```python
from build123d import *

# Parameters (mm, degrees)
PAD004_DEPTH    = 30
FILLET002_R     = 5
FILLET003_R     = 5
CHAMFER002_SIZE = 1


with BuildPart() as part:
    # Sketch006 → Pad004 (new body)
    with BuildSketch(Plane.YZ):
        Polygon((0, 0), (0, 80), (-5, 80), (-5, 121.25), (32.5, 121.25), (32.5, 116.25), (2.5, 116.25), (2.5, -36.25), (32.5, -36.25), (32.5, -41.25), (-5, -41.25), (-5, 0), align=None)
    extrude(amount=PAD004_DEPTH)

    # Fillet002
    fillet002_edges = [part.edges().sort_by_distance(p)[0] for p in [
        (0, 32.5, 118.75),
        (30, 32.5, 118.75),
        (0, 32.5, -38.75),
        (30, 32.5, -38.75),
    ]]
    fillet(fillet002_edges, radius=FILLET002_R)

    # Fillet003
    fillet003_edges = [part.edges().sort_by_distance(p)[0] for p in [
        (15, -5, 121.25),
        (15, -5, -41.25),
    ]]
    fillet(fillet003_edges, radius=FILLET003_R)

    # Chamfer002
    chamfer002_edges = [part.edges().sort_by_distance(p)[0] for p in [
        (30, 2.5, 40),
        (0, 2.5, 40),
        (15, 32.5, 116.25),
        (15, 32.5, -36.25),
        (15, 32.5, -41.25),
        (15, 32.5, 121.25),
        (15, -5, 80),
        (15, -5, 0),
    ]]
    chamfer(chamfer002_edges, length=CHAMFER002_SIZE)


solid = part.part
```
CAD build for the part. Positions are in the model's coordinates, mm. A direction names the side the tool comes from. Round coordinates to 2 decimals unless told otherwise and drop trailing zeros. Loops run counter-clockwise (first coordinate to the right, second up) from the corner with the lowest first, then second, coordinate; pieces in that order, holes last. Notation, with made-up numbers: (-15, 35) - (10, 35) arc R25 cw to (10, 54) - close; hole circle Ø6 at (-9, 1). An arc over 180 degrees is marked (long way). Return JSON: item names as keys, results as strings. Group by question number.
Q1. Tool access for faces 4 (the face through (1.95, 30.49, 116.52)), 5 (the face through (15, 17, -36.25)), 6 (the face through (1.937, 30.496, 120.965)), 7 (the face through (15, -5, 98)), 8 (the face through (15, 0, 39)): list every direction of +Z, -Z, +X, -X, +Y, -Y with a clear straight run to the whole face (end or side of a thin tool).
Q2. Drill centre lines: line 1 along Z through (x, y) = (21.5, 17.5); line 2 along Y through (x, z) = (24.5, 67.5); line 3 along Y through (x, z) = (11.5, -7.5). Where is each one in solid material? Low to high. Write a range as [from, to].
Q3. Flat gauge pins, fed straight in: pin 1 Ø8 at (x, z) = (13, 51.5) entering from -Y; pin 2 Ø8 at (y, z) = (8.5, 9.5) entering from +X; pin 3 Ø10 at (x, z) = (22, 9.5) entering from +Y; pin 4 Ø4.5 at (x, y) = (12.5, -2.5) entering from +Z. Where does each tip first touch, or does it go through?
Q4. Band-saw the part on A-A on y = 7. Give the cut face in (x, z).
Q5. Band-saw the part on B-B on x = 20.5. Give the cut face in (y, z).
Q6. Band-saw the part on D-D on z = 6.5. Give the cut face in (x, y).
Q7. Two-plate mould, pull along Z, no slides. Class faces 1 (the face through (1.937, 30.496, -36.535)), 2 (the face through (15, 32.5, -39)), 3 (the face through (0.27, -3.05, 119.24)): +Z half, -Z half, draft (parallel to the pull), parting line (faces both ways), or undercut.
Q8. Band-saw the part on C-C on z = 84. Give the cut face in (x, y).
Solutions:
{
 "1": {"face 4": "-X, +Y", "face 5": "+X, -X, +Y", "face 6": "+Z, -X, +Y", "face 7": "+Z, -Z, +X, -X, -Y", "face 8": "+X, -X, -Y"},
 "2": {"line 1": "z = [-41.25, -36.25], [116.25, 121.25]", "line 2": "y = [0, 2.5]", "line 3": "y = [-5, 2.5]"},
 "3": {"pin 1": "stops at y = 0", "pin 2": "passes through", "pin 3": "stops at y = 2.5", "pin 4": "stops at z = 121.24"},
 "4": {"outline": "(0, -40.25) - (1, -41.25) - (29, -41.25) - (30, -40.25) - (30, -37.25) - (29, -36.25) - (1, -36.25) - (0, -37.25) - close; (0, 117.25) - (1, 116.25) - (29, 116.25) - (30, 117.25) - (30, 120.25) - (29, 121.25) - (1, 121.25) - (0, 120.25) - close"},
 "5": {"outline": "(-5, -36.25) arc R5 ccw to (0, -41.25) - (31.5, -41.25) - (32.5, -40.25) - (32.5, -37.25) - (31.5, -36.25) - (2.5, -36.25) - (2.5, 116.25) - (31.5, 116.25) - (32.5, 117.25) - (32.5, 120.25) - (31.5, 121.25) - (0, 121.25) arc R5 ccw to (-5, 116.25) - (-5, 81) - (-4, 80) - (0, 80) - (0, 0) - (-4, 0) - (-5, -1) - close"},
 "6": {"outline": "(0, 0) - (30, 0) - (30, 1.5) - (29, 2.5) - (1, 2.5) - (0, 1.5) - close"},
 "7": {"face 1": "undercut", "face 2": "draft", "face 3": "+Z half"},
 "8": {"outline": "(0, -4) - (1, -5) - (29, -5) - (30, -4) - (30, 1.5) - (29, 2.5) - (1, 2.5) - (0, 1.5) - close"}
}
